```python
from build123d import *

# Parameters (mm, degrees)
F0_W     = 1100
F0_H     = 1100
F1_DEPTH = 25
F2_W     = 1000
F2_H     = 1000
F2_W_2   = 950
F2_H_2   = 950
F3_DEPTH = 25


with BuildPart() as f1:
    # F0 (on Top) → F1 (new body)
    with BuildSketch(Plane.XY):
        Rectangle(F0_W, F0_H)
    extrude(amount=F1_DEPTH)

    # F2 (on face) → F3 (join)
    with BuildSketch(Plane(origin=(0, 0, 0), x_dir=(1, 0, 0), z_dir=(0, 0, -1))):
        Rectangle(F2_W, F2_H)
        Rectangle(F2_W_2, F2_H_2, mode=Mode.SUBTRACT)
    extrude(amount=F3_DEPTH)


solid = f1.part
```
Verification items for the finished model (mm, model axes). A direction names the side the tool comes from. Give positions to 0.01 mm unless a question says otherwise; leave off trailing zeros. Write each loop counter-clockwise with the first axis right and the second up, starting at its lowest first coordinate (ties: lowest second). Pieces come first, ordered by that corner, then holes. Notation, with made-up numbers: M 15.5,-7 L 73.5,-7 A21 cw 73.5,21 Z; hole C -32.5,4.5 d4. An arc over 180 degrees is marked long. One line per question, with ' | ' between items.
1) Set-up check for faces 4 (the flat face through (-500, 7, -12)), 5 (the flat face through (-7, -475, -12)), 6 (the flat face through (-7, 500, -12)): record each of +Z, -Z, +X, -X, +Y, -Y from which the full face is reachable in a straight line by a thin tool's end or side.
Result:
face 4: -Z, -X, +Y, -Y | face 5: -Z | face 6: -Z, +X, -X, +Y
2) Section check A-A on z = -11.5. Enter the section's corners in (x, y), plus the area to 3 significant figures.
Result:
outline: M -500,-500 L 500,-500 L 500,500 L -500,500 Z; hole M -475,-475 L 475,-475 L 475,475 L -475,475 Z | area: 97,500 mm2
3) Gauge pin test, flat ends, axial feed: pin 1 Ø20 at (x, z) = (-187, -16.5) entering from +Y; pin 2 Ø7.5 at (x, z) = (205.5, -14) entering from -Y; pin 3 Ø1.5 at (x, y) = (153.5, -331) entering from -Z. Record the tip position at first contact, or that the pin passes through.
Result:
pin 1: stops at y = 500 | pin 2: stops at y = -500 | pin 3: stops at z = 0
4) Section check B-B on y = 433.5. Enter the section's corners in (x, z), plus the area to 4 significant figures.
Result:
outline: M -550,0 L -500,0 L -500,-25 L -475,-25 L -475,0 L 475,0 L 475,-25 L 500,-25 L 500,0 L 550,0 L 550,25 L -550,25 Z | area: 28,750 mm2
5) Mould release check, pull along X, two halves, no side actions. Record for faces 1 (the flat face through (475, 7, -12)), 2 (the flat face through (-7, -500, -12)), 3 (the flat face through (-550, -8, 12)): released by +X, released by -X, zero draft, split by the parting line, or undercut.
Result:
face 1: undercut | face 2: zero draft | face 3: released by -X
6) Thickness scan on line 1 along Y through (x, z) = (-46, -8); line 2 along Z through (x, y) = (251, -351). Record the ranges inside material, lowest first. Write a range as [from, to].
Result:
line 1: y = [-500, -475], [475, 500] | line 2: z = [0, 25]
